from build123d import *


with BuildPart() as part:
    # Esquisse1 → Révolution1 (revolve)
    with BuildSketch(Plane.XY, mode=Mode.PRIVATE) as r_volution1_sk:
        Polygon((-13.941052428, 17), (-13.941052428, 20.25), (-13.441052428, 20.75), (-3.941052428, 20.75), (-3.941052428, 21.75), (-3.691052428, 22), (-1.191052428, 22), (-0.941052428, 21.75), (-0.941052428, 19.5), (5.192922168, 19.5), (6.058947572, 19), (6.058947572, 17), (5.558947572, 16.5), (-13.441052428, 16.5), align=None)
    revolve(r_volution1_sk.sketch.rotate(Axis((0, 0, 0), (1, 0, 0)), 90), axis=Axis((0, 0, 0), (1, 0, 0)))  # turned: the seam where the file's is


solid = part.part
Geometry check sheet. Reference: the model listing, model coordinates, mm. A direction names the side the tool comes from. Give positions to 0.01 mm unless a question says otherwise; leave off trailing zeros. Write each loop counter-clockwise with the first axis right and the second up, starting at its lowest first coordinate (ties: lowest second). Pieces come first, ordered by that corner, then holes.
1) Go/stop test with flat-tipped pins: pin 1 Ø6 at (y, z) = (9.5, -8.5) entering from +X; pin 2 Ø2 at (x, y) = (-10.5, 10) entering from +Z; pin 3 Ø5 at (x, y) = (-11.5, 16) entering from +Z; pin 4 Ø12 at (x, y) = (0, -6.5) entering from -Z. Record where each tip stops, or that it passes through.
Values follow:
pin 1: passes through
pin 2: stops at z = 18.7
pin 3: stops at z = 15.76
pin 4: stops at z = -21.99
2) Cross-section at A-A (y = 0). Record the boundary of the cut face in (x, z), plus the area to 3 significant figures.
Values follow:
outline: (-13.94, -20.25) - (-13.44, -20.75) - (-3.94, -20.75) - (-3.94, -21.75) - (-3.69, -22) - (-1.19, -22) - (-0.94, -21.75) - (-0.94, -19.5) - (5.19, -19.5) - (6.06, -19) - (6.06, -17) - (5.56, -16.5) - (-13.44, -16.5) - (-13.94, -17) - close; (-13.94, 17) - (-13.44, 16.5) - (5.56, 16.5) - (6.06, 17) - (6.06, 19) - (5.19, 19.5) - (-0.94, 19.5) - (-0.94, 21.75) - (-1.19, 22) - (-3.69, 22) - (-3.94, 21.75) - (-3.94, 20.75) - (-13.44, 20.75) - (-13.94, 20.25) - close
area: 159 mm2
3) Set-up check for faces 1 (the face through (6.059, 10, -14)), 2 (the face through (2.169, -19.334, -2.539)), 3 (the face through (-3.941, 11, -18)): record each of +Z, -Z, +X, -X, +Y, -Y from which the full face is reachable in a straight line by a thin tool's end or side.
Values follow:
face 1: +Z, -Z, +X, +Y, -Y
face 2: +X
face 3: -X
4) Thickness scan on line 1 (Y direction, x = -5.5, z = 0); line 2 (Y direction, x = 3, z = 10); line 3 (X direction, y = 9, z = -19). Record the ranges inside material, lowest first.
Values follow:
line 1: y = -20.75 to -16.5, 16.5 to 20.75
line 2: y = -16.74 to -13.12, 13.12 to 16.74
line 3: x = -3.94 to -0.94
5) Release check for a two-part mould opening along Z. For faces 4 (the face through (-4.074, -4.956, 15.738)), 5 (the face through (-8.6, -6.2, 19.8)), 6 (the face through (-13.941, -17, 5)) record: released by +Z, released by -Z, zero draft, split by the parting line, or undercut.
Values follow:
face 4: undercut
face 5: split by the parting line
face 6: zero draft
6) Cross-section at D-D (x = -2.5). Record the boundary of the cut face in (y, z).
Values follow:
outline: circle Ø44 at (0, 0); hole circle Ø33 at (0, 0)
7) Cross-section at C-C (x = 3.25). Record the boundary of the cut face in (y, z), plus the area to 3 significant figures.
Values follow:
outline: circle Ø39 at (0, 0); hole circle Ø33 at (0, 0)
area: 339 mm2
